Geometry check sheet. Reference: the model listing, model coordinates, mm. Round coordinates to 2 decimals unless told otherwise and drop trailing zeros. Write each loop counter-clockwise with the first axis right and the second up, starting at its lowest first coordinate (ties: lowest second). Pieces come first, ordered by that corner, then holes. Notation, with made-up numbers: (-0.75, 10) -> (39.25, 10) arc R11 ccw to (39.25, 23) -> close; hole circle Ø6 at (-15, 29.25). An arc over 180 degrees is marked (long way). One line per question, with ' | ' between items.
```python
from build123d import *

# Parameters (mm, degrees)
SKETCH2_W            = 39.4
SKETCH2_H            = 23.4
HATCH_PLATE_DEPTH    = 2.4
SKETCH3_W            = 7
SKETCH3_H            = 14
SKETCH3_R            = 1.55
DRIVE_ARM_D3P1_DEPTH = 2.4


with BuildPart() as part:
    # Sketch2 → Hatch_plate (new body)
    with BuildSketch(Plane.XY):
        Rectangle(SKETCH2_W, SKETCH2_H)
    extrude(amount=HATCH_PLATE_DEPTH)

    # Sketch3 → Drive_arm_D3p1 (add)
    with BuildSketch(Plane.XY):
        with Locations((0, 18)):
            Rectangle(SKETCH3_W, SKETCH3_H)
        with Locations((0, 20.5)):
            Circle(SKETCH3_R, mode=Mode.SUBTRACT)
    extrude(amount=DRIVE_ARM_D3P1_DEPTH)


solid = part.part
```
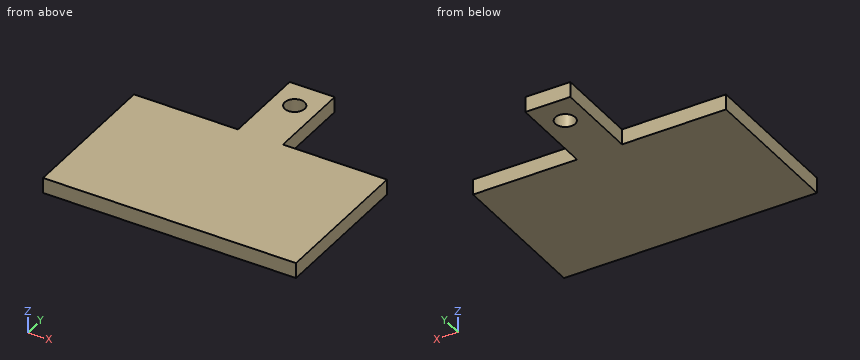
(1) Sectioned sample at B-B on x = 0. Record the cut outline in (y, z), then the cut area to 3 significant figures.
Resolved:
outline: (-11.7, 0) -> (18.95, 0) -> (18.95, 2.4) -> (-11.7, 2.4) -> close; (22.05, 0) -> (25, 0) -> (25, 2.4) -> (22.05, 2.4) -> close | area: 80.6 mm2
(2) Go/stop test with flat-tipped pins: pin 1 (0.7 mm diameter, centred on y = 20, z = 1.5, fed in from +X); pin 2 (0.7 mm diameter, centred on x = 9, z = 1, fed in from +Y). Record where each tip stops, or that it passes through.
Resolved:
pin 1: stops at x = 3.5 | pin 2: stops at y = 11.7
(3) Sectioned sample at C-C on y = 20.5. Record the cut outline in (x, z), then the cut area to 3 significant figures.
Resolved:
outline: (-3.5, 0) -> (-1.55, 0) -> (-1.55, 2.4) -> (-3.5, 2.4) -> close; (1.55, 0) -> (3.5, 0) -> (3.5, 2.4) -> (1.55, 2.4) -> close | area: 9.36 mm2
(4) Sectioned sample at A-A on z = 0.95. Record the cut outline in (x, y).
Resolved:
outline: (-19.7, -11.7) -> (19.7, -11.7) -> (19.7, 11.7) -> (3.5, 11.7) -> (3.5, 25) -> (-3.5, 25) -> (-3.5, 11.7) -> (-19.7, 11.7) -> close; hole circle Ø3.1 at (0, 20.5)
(5) Material ranges on line 1 (Y direction, x = 0, z = 1.3); line 2 (Y direction, x = -12, z = 1.55); line 3 (X direction, y = 19.5, z = 1.35), recorded low to high.
Resolved:
line 1: y = -11.7 to 18.95, 22.05 to 25 | line 2: y = -11.7 to 11.7 | line 3: x = -3.5 to -1.18, 1.18 to 3.5
(6) Sectioned sample at D-D on x = -10. Record the cut outline in (y, z).
Resolved:
outline: (-11.7, 0) -> (11.7, 0) -> (11.7, 2.4) -> (-11.7, 2.4) -> close
